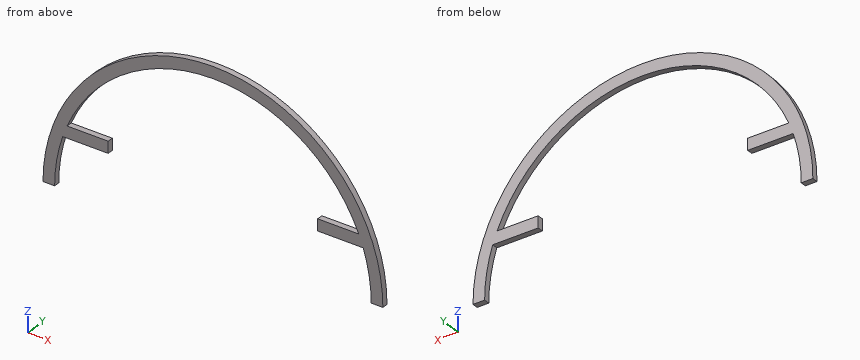
```python
from build123d import *

# Parameters (mm, degrees)
BOSS_EXTRUDE1_DEPTH = 3.175


with BuildPart() as part:
    # Sketch1 → Boss-Extrude1 (new body)
    with BuildSketch(Plane(origin=(0, 0, 0), x_dir=(1, 0, 0), z_dir=(0, 1, 0))):
        with BuildLine():
            Line((-57.15, -27.220431682), (-81.957901993, -27.220431682))
            ThreePointArc((-81.957901993, -27.220431682), (-80.82536417, -30.418910347), (-79.568057138, -33.570431682))
            Line((-79.568057138, -33.570431682), (-57.15, -33.570431682))
            Line((-57.15, -33.570431682), (-57.15, -27.220431682))
        make_face()
        with BuildLine():
            Line((-86.36, 0), (-92.71, 0))
            ThreePointArc((-92.71, 0), (0, -92.71), (92.71, 0))
            Line((92.71, 0), (86.36, 0))
            ThreePointArc((86.36, 0), (85.252372448, -13.787044351), (81.957901993, -27.220431682))
            Line((81.957901993, -27.220431682), (81.957901993, -33.570431682))
            Line((81.957901993, -33.570431682), (79.568057138, -33.570431682))
            ThreePointArc((79.568057138, -33.570431682), (0, -86.36), (-79.568057138, -33.570431682))
            Line((-79.568057138, -33.570431682), (-81.957901993, -33.570431682))
            Line((-81.957901993, -33.570431682), (-81.957901993, -27.220431682))
            ThreePointArc((-81.957901993, -27.220431682), (-85.252372448, -13.787044351), (-86.36, 0))
        make_face()
        with BuildLine():
            ThreePointArc((-79.568057138, -33.570431682), (-80.82536417, -30.418910347), (-81.957901993, -27.220431682))
            Line((-81.957901993, -27.220431682), (-81.957901993, -33.570431682))
            Line((-81.957901993, -33.570431682), (-79.568057138, -33.570431682))
        make_face()
        with BuildLine():
            Line((81.957901993, -33.570431682), (81.957901993, -27.220431682))
            ThreePointArc((81.957901993, -27.220431682), (80.82536417, -30.418910347), (79.568057138, -33.570431682))
            Line((79.568057138, -33.570431682), (81.957901993, -33.570431682))
        make_face()
        with BuildLine():
            ThreePointArc((79.568057138, -33.570431682), (80.82536417, -30.418910347), (81.957901993, -27.220431682))
            Line((81.957901993, -27.220431682), (57.15, -27.220431682))
            Line((57.15, -27.220431682), (57.15, -33.570431682))
            Line((57.15, -33.570431682), (79.568057138, -33.570431682))
        make_face()
    extrude(amount=BOSS_EXTRUDE1_DEPTH)


solid = part.part
```
Verification items for the finished model (mm, model axes). Round coordinates to 2 decimals unless told otherwise and drop trailing zeros. Write each loop counter-clockwise with the first axis right and the second up, starting at its lowest first coordinate (ties: lowest second). Pieces come first, ordered by that corner, then holes.
1. Scan lines: L1, parallel to X at y = 1.35, z = 75.5; L2, parallel to X at y = 2, z = 70.5; L3, parallel to Z at x = 79.5, y = 0.3. Record each from-to range of solid material in increasing order.
2. Section check A-A on z = 77.5. Enter the section's corners in (x, y) (3 decimals), plus the area to 3 significant figures.
3. Section check C-C on x = -65.5. Enter the section's corners in (y, z) (3 decimals).
4. Section check D-D on x = 0. Enter the section's corners in (y, z) (3 decimals).
5. Section check B-B on y = 2.6. Enter the section's corners in (x, z).
6. Gauge pin test, flat ends, axial feed: P1, Ø1, axis at y = 1.5, z = 29.5, coming from the +X side; P2, Ø10, axis at x = -59.5, z = 43.5, coming from the +Y side; P3, Ø1, axis at x = -73, y = 1.5, coming from the +Z side; P4, Ø1, axis at y = 1.5, z = 18, coming from the +X side. Record the tip position at first contact, or that the pin passes through.
Answer:
1. L1: x = -53.8 to -41.93, 41.93 to 53.8
1. L2: x = -60.21 to -49.88, 49.88 to 60.21
1. L3: z = 27.22 to 33.57, 33.73 to 47.7
2. outline: (-50.881, 0) - (-38.102, 0) - (-38.102, 3.175) - (-50.881, 3.175) - close; (38.102, 0) - (50.881, 0) - (50.881, 3.175) - (38.102, 3.175) - close
2. area: 81.1 mm2
3. outline: (0, 27.22) - (3.175, 27.22) - (3.175, 33.57) - (0, 33.57) - close; (0, 56.283) - (3.175, 56.283) - (3.175, 65.612) - (0, 65.612) - close
4. outline: (0, 86.36) - (3.175, 86.36) - (3.175, 92.71) - (0, 92.71) - close
5. outline: (-92.71, 0) - (-86.36, 0) arc R86.36 cw to (-81.96, 27.22) - (-57.15, 27.22) - (-57.15, 33.57) - (-79.57, 33.57) arc R86.36 cw to (79.57, 33.57) - (57.15, 33.57) - (57.15, 27.22) - (81.96, 27.22) arc R86.36 cw to (86.36, 0) - (92.71, 0) arc R92.71 ccw to start
6. P1: stops at x = 88.06
6. P2: passes through
6. P3: stops at z = 57.78
6. P4: stops at x = 91.04
